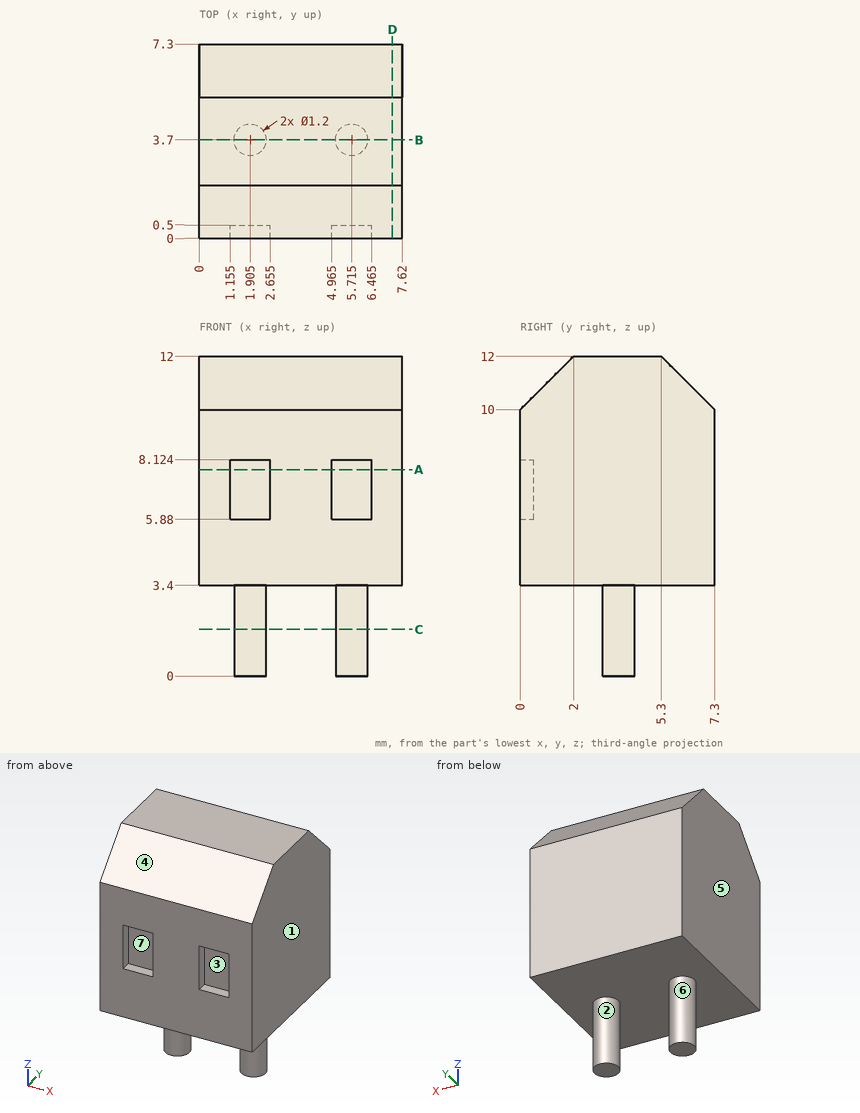
Here's the drawing with two shaded views (mm, measured from the low corner). I have some questions. A direction names the side the tool comes from. Give positions to 0.01 mm unless a question says otherwise; leave off trailing zeros. Loops run counter-clockwise (first coordinate to the right, second up) from the corner with the lowest first, then second, coordinate; pieces in that order, holes last. Notation, with made-up numbers: (15, 17) - (73, 17) arc R26 ccw to (73, 44) - close; hole circle Ø1 at (-5.5, 56.25). An arc over 180 degrees is marked (long way). Return JSON: item names as keys, results as strings.
1. If I drill on line 1 (Z direction, x = 5.5, y = 5); line 2 (Z direction, x = 1, y = 6.75); line 3 (Y direction, x = 6, z = 11.25), over which ranges is the centre line in solid material (lowest first)?
Output values:
{"line 1": "z = 3.4 to 12", "line 2": "z = 3.4 to 10.55", "line 3": "y = 1.25 to 6.05"}
2. For the marked faces 1, 2 and 3, which set-ups out of +Z, -Z, +X, -X, +Y, -Y let a thin tool reach every point of the face, with its end or its side?
Output values:
{"face 1": "+Z, -Z, +X, +Y, -Y", "face 2": "-Z", "face 3": "-Y"}
3. I'm going to push a flat-ended pin straight in: pin 1 Ø0.6 at (x, y) = (6, 0.5) entering from +Z. Where does the tip first touch, or does it pass through?
Output values:
{"pin 1": "stops at z = 10.8"}
4. I want a section at A-A on z = 7.75. Please give me the cut outline in (x, y) (1 decimal).
Output values:
{"outline": "(0, 0) - (1.2, 0) - (1.2, 0.5) - (2.7, 0.5) - (2.7, 0) - (5, 0) - (5, 0.5) - (6.5, 0.5) - (6.5, 0) - (7.6, 0) - (7.6, 7.3) - (0, 7.3) - close"}
5. I want a section at C-C on z = 1.75. Please give me the cut outline in (x, y) (1 decimal).
Output values:
{"outline": "circle Ø1.2 at (1.9, 3.7); circle Ø1.2 at (5.7, 3.7)"}
6. I want a section at D-D on x = 7.25. Please give me the cut outline in (y, z), and give its area (3 significant figures).
Output values:
{"outline": "(0, 3.4) - (7.3, 3.4) - (7.3, 10) - (5.3, 12) - (2, 12) - (0, 10) - close", "area": "58.8 mm²"}
7. We'd pull the mould along X, two halves only. Please class the marked faces 4, 5, 6 and 7: +X half, -X half, draft (parallel to the pull), parting line (faces both ways), or undercut.
Output values:
{"face 4": "draft", "face 5": "-X half", "face 6": "undercut", "face 7": "undercut"}
8. I want a section at B-B on y = 3.7. Please give me the cut outline in (x, z) (1 decimal), and give its area (3 significant figures).
Output values:
{"outline": "(0, 3.4) - (1.3, 3.4) - (1.3, 0) - (2.5, 0) - (2.5, 3.4) - (5.1, 3.4) - (5.1, 0) - (6.3, 0) - (6.3, 3.4) - (7.6, 3.4) - (7.6, 12) - (0, 12) - close", "area": "73.7 mm²"}
